Verification items for the finished model (mm, model axes). A direction names the side the tool comes from. Give positions to 0.01 mm unless a question says otherwise; leave off trailing zeros. Loops run counter-clockwise (first coordinate to the right, second up) from the corner with the lowest first, then second, coordinate; pieces in that order, holes last. Notation, with made-up numbers: (80.25, 24) -> (131.25, 24) arc R18 ccw to (131.25, 30) -> close; hole circle Ø1 at (-20, -27). An arc over 180 degrees is marked (long way). Answer in a Markdown table with one row per item. Add a question column.
Q1. Section check D-D on y = 7. Enter the section's corners in (x, z), and give its area (3 significant figures).
Q2. Set-up check for faces 4 (the face through (6, -19, 20)), 5 (the face through (-18, 0, 21)): record each of +Z, -Z, +X, -X, +Y, -Y from which the full face is reachable in a straight line by a thin tool's end or side.
Q3. Material ranges on probe 1 along X at (y, z) = (11, 38.5); probe 2 along Z at (x, y) = (0, 19.5), recorded low to high.
Q4. Gauge pin test, flat ends, axial feed: P1, Ø6, axis at x = 8.5, y = -11, coming from the +Z side; P2, Ø19, axis at x = 0, z = 20, coming from the -Y side; P3, Ø9.5, axis at x = 0, z = 20, coming from the -Y side. Record the tip position at first contact, or that the pin passes through.
Q5. Release check for a two-part mould opening along Y. For faces 1 (the face through (5, 20, 15)), 2 (the face through (18, 0, 21)), 3 (the face through (6, 19, 20)) record: pulls with the +Y half, pulls with the -Y half, needs draft (parallel to the pull), parting line crosses it, or undercut.
Q6. Section check A-A on z = 20. Enter the section's corners in (x, y), and give its area (3 significant figures).
Q7. Section check B-B on z = 10.5. Enter the section's corners in (x, y).
Q8. Section check C-C on x = 2. Enter the section's corners in (y, z).
```python
from build123d import *

# Parameters (mm, degrees)
SKETCH1_W           = 40
SKETCH1_H           = 40
BOSS_EXTRUDE1_DEPTH = 40
SHELL1_T            = -2
SKETCH2_R           = 6
CUT_EXTRUDE1_DEPTH  = 40


with BuildPart() as part:
    # Sketch1 → Boss-Extrude1 (new body)
    with BuildSketch(Plane(origin=(0, 0, 0), x_dir=(0, 1, 0), z_dir=(0, 0, 1))):
        Rectangle(SKETCH1_W, SKETCH1_H)
    extrude(amount=BOSS_EXTRUDE1_DEPTH)

    # Shell1
    shell1_openings = [part.faces().sort_by_distance(p)[0] for p in [
        (0, 0, 40),
    ]]
    offset(amount=SHELL1_T, openings=shell1_openings, kind=Kind.INTERSECTION)

    # Sketch2 → Cut-Extrude1 (cut)
    with BuildSketch(Plane(origin=(0, 20, 0), x_dir=(-1, 0, 0), z_dir=(0, 1, 0))):
        with Locations((0, 20)):
            Circle(SKETCH2_R)
    extrude(amount=-CUT_EXTRUDE1_DEPTH, mode=Mode.SUBTRACT)


solid = part.part
```
Taken from the geometry:
| question | item | result |
|---|---|---|
| 1 | outline | (-20, 0) -> (20, 0) -> (20, 40) -> (18, 40) -> (18, 2) -> (-18, 2) -> (-18, 40) -> (-20, 40) -> close |
| 1 | area | 232 mm² |
| 2 | face 4 | +Y, -Y |
| 2 | face 5 | +Z |
| 3 | probe 1 | x = -20 to -18, 18 to 20 |
| 3 | probe 2 | z = 0 to 14, 26 to 40 |
| 4 | P1 | stops at z = 2 |
| 4 | P2 | stops at y = -20 |
| 4 | P3 | passes through |
| 5 | face 1 | pulls with the +Y half |
| 5 | face 2 | undercut |
| 5 | face 3 | needs draft |
| 6 | outline | (-20, -20) -> (-6, -20) -> (-6, -18) -> (-18, -18) -> (-18, 18) -> (-6, 18) -> (-6, 20) -> (-20, 20) -> close; (6, -20) -> (20, -20) -> (20, 20) -> (6, 20) -> (6, 18) -> (18, 18) -> (18, -18) -> (6, -18) -> close |
| 6 | area | 256 mm² |
| 7 | outline | (-20, -20) -> (20, -20) -> (20, 20) -> (-20, 20) -> close; hole (-18, -18) -> (18, -18) -> (18, 18) -> (-18, 18) -> close |
| 8 | outline | (-20, 0) -> (20, 0) -> (20, 14.34) -> (18, 14.34) -> (18, 2) -> (-18, 2) -> (-18, 14.34) -> (-20, 14.34) -> close; (-20, 25.66) -> (-18, 25.66) -> (-18, 40) -> (-20, 40) -> close; (18, 25.66) -> (20, 25.66) -> (20, 40) -> (18, 40) -> close |
